Autodesk Inventor part; units mm, degrees
ref_plane "YZ Plane" through (0, 0, 0) normal (1, 0, 0) x (0, 1, 0)
ref_plane "XZ Plane" through (0, 0, 0) normal (0, 1, 0) x (-1, 0, 0)
ref_plane "XY Plane" through (0, 0, 0) normal (0, 0, 1) x (1, 0, 0)
sketch "Sketch1" plane through (0, 0, 0) normal (0, 0, 1) x (1, 0, 0)
  line L0 (-5.5426, -7.3901) -> (-9.1713, 1.105)
  line L1 (-9.1713, 1.105) -> (-3.6287, 8.495)
  line L2 (-3.6287, 8.495) -> (5.5426, 7.3901)
  line L3 (5.5426, 7.3901) -> (9.1713, -1.105)
  line L4 (9.1713, -1.105) -> (3.6287, -8.495)
  line L5 (3.6287, -8.495) -> (-5.5426, -7.3901)
  point P0 (0, 0)
  point P1 (0, 0)
  dimension "d0" = 16
extrude "Extrusion1" add sketch "Sketch1" along normal blind 13
sketch "Sketch2" plane through (0, 0, 13) normal (0, 0, 1) x (1, 0, 0)
  point P0 (0, 0)
hole "Hole1" at (0, 0, 13) direction (0, 0, -1) diameter 11.835 depth 9
sketch "Sketch3" plane through (0, 0, 0) normal (0, 0, -1) x (-1, 0, 0)
  point P0 (0, 0)
hole "Hole2" at (0, 0, 0) direction (0, 0, 1) diameter 10 depth 9
properties part number "HUDSON-1-108"
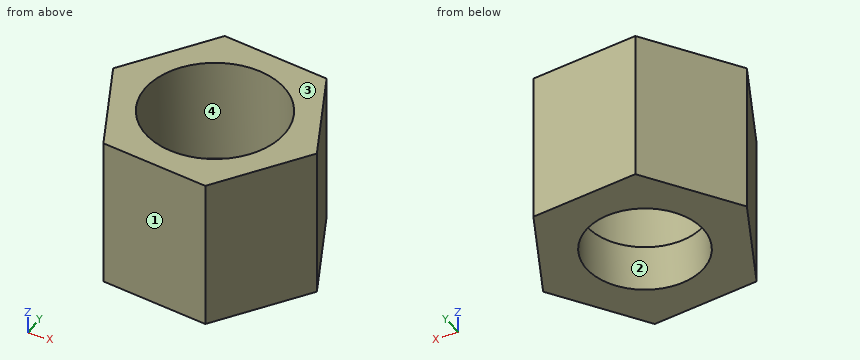
Input: part model. Units: mm. Frame: model coordinates. Face numbers are marked on the shaded views. Give positions to 0.01 mm unless a question says otherwise; leave off trailing zeros. Order: outer loops, then holes, each group sorted by start corner. A loop starts at its lowest first (then second) coordinate and runs counter-clockwise, first axis right, second up. Notation, with made-up numbers: M -4,19.25 L 13,19.25 A26 ccw 13,57.25 Z; hole C 13.5,24 d5. An arc over 180 degrees is marked long. Return JSON: item names as keys, results as strings.
1) Section query A-A on z = 10. Output: boundary loops of the cut face in (x, y) (1 decimal).
Taken from the geometry:
{"outline": "M -9.2,1.1 L -5.5,-7.4 L 3.6,-8.5 L 9.2,-1.1 L 5.5,7.4 L -3.6,8.5 Z; hole C 0,0 d11.8"}
2) Section query C-C on y = 0. Output: boundary loops of the cut face in (x, z), and give its area (3 significant figures).
Taken from the geometry:
{"outline": "M -8.7,0 L -5,0 L -5,4 L -5.92,4 L -5.92,13 L -8.7,13 Z; M 5,0 L 8.7,0 L 8.7,13 L 5.92,13 L 5.92,4 L 5,4 Z", "area": "79.7 mm2"}
3) Section query D-D on z = 2.5. Output: boundary loops of the cut face in (x, y) (3 decimals).
Taken from the geometry:
{"outline": "M -9.171,1.105 L -5.543,-7.39 L 3.629,-8.495 L 9.171,-1.105 L 5.543,7.39 L -3.629,8.495 Z; hole C 0,0 d10"}
4) Mould query, pull axis Y, two halves, no side actions, for the marked faces 1, 2, 3 and 4. Classes: released by +Y, released by -Y, zero draft, split by the parting line, or undercut.
Taken from the geometry:
{"face 1": "released by -Y", "face 2": "undercut", "face 3": "zero draft", "face 4": "undercut"}
5) Section query B-B on x = 0. Output: boundary loops of the cut face in (y, z).
Taken from the geometry:
{"outline": "M -8.06,0 L -5,0 L -5,4 L -5.92,4 L -5.92,13 L -8.06,13 Z; M 5,0 L 8.06,0 L 8.06,13 L 5.92,13 L 5.92,4 L 5,4 Z"}
6) Line query: L1, parallel to X at y = 0, z = 6.5; L2, parallel to Y at x = -5.25, z = 7.25; L3, parallel to Y at x = 4.25, z = 9.5. Output: solid intervals per line, ascending. Write a range as [from, to].
Taken from the geometry:
{"L1": "x = [-8.7, -5.92], [5.92, 8.7]", "L2": "y = [-7.43, -2.73], [2.73, 6.33]", "L3": "y = [-7.67, -4.12], [4.12, 7.55]"}
7) Contact query for flat-ended pins moving along their axis: pin 1 (6 mm diameter, centred on x = -2, z = 6, fed in from -Y); pin 2 (3 mm diameter, centred on x = -4, z = 1.5, fed in from -Y); pin 3 (2 mm diameter, centred on x = 0.5, z = 10, fed in from +Y). Output: stop coordinate, or through.
Taken from the geometry:
{"pin 1": "stops at y = -8.18", "pin 2": "stops at y = -7.76", "pin 3": "stops at y = 8.12"}
